```python
from build123d import *

# Parameters (mm, degrees)
IZIM1_R                     = 2
IZIM1_R_2                   = 1.5
Y_KSEKLIK_EKSTR_ZYON1_DEPTH = 1.7
IZIM2_R                     = 2
Y_KSEKLIK_EKSTR_ZYON2_DEPTH = 2.6
IZIM3_W                     = 4.100055298
IZIM3_H                     = 6.25
Y_KSEKLIK_EKSTR_ZYON3_DEPTH = 8.5
IZIM4_W                     = 5.8
IZIM4_H                     = 6.25
Y_KSEKLIK_EKSTR_ZYON4_DEPTH = 0.6
Y_KSEKLIK_EKSTR_ZYON6_DEPTH = 2.54
IZIM6_W                     = 19.85
IZIM6_H                     = 1.7
Y_KSEKLIK_EKSTR_ZYON7_DEPTH = 0.01
IZIM7_W                     = 6.75
IZIM7_H                     = 0.75
KES_EKSTR_ZYON1_DEPTH       = 5.9
KES_EKSTR_ZYON1_DEPTH_BACK  = 0.1
IZIM8_W                     = 0.664910116
IZIM8_H                     = 0.664910116
IZIM11_W                    = 0.65
IZIM11_H                    = 0.6
Y_KSEKLIK_EKSTR_ZYON8_DEPTH = 1
Y_KSEKLIK_EKSTR_ZYON9_DEPTH = 1.5


with BuildPart() as part:
    # Çizim1 → Yükseklik-Ekstrüzyon1 (new body)
    with BuildSketch(Plane.XY):
        with BuildLine():
            Line((-9.925, -11.575), (9.925, -11.575))
            Line((9.925, -11.575), (9.925, 4.275))
            ThreePointArc((9.925, 4.275), (13.575, 7.925), (9.925, 11.575))
            Line((9.925, 11.575), (-9.925, 11.575))
            ThreePointArc((-9.925, 11.575), (-13.575, 7.925), (-9.925, 4.275))
            Line((-9.925, 4.275), (-9.925, -11.575))
        make_face()
        with Locations((9.925, 7.925)):
            Circle(IZIM1_R, mode=Mode.SUBTRACT)
        with Locations((-9.925, 7.925)):
            Circle(IZIM1_R, mode=Mode.SUBTRACT)
        with Locations((7.925, -2.575)):
            Circle(IZIM1_R_2, mode=Mode.SUBTRACT)
        with Locations((-7.925, -2.575)):
            Circle(IZIM1_R_2, mode=Mode.SUBTRACT)
    extrude(amount=Y_KSEKLIK_EKSTR_ZYON1_DEPTH)

    # Çizim2 → Yükseklik-Ekstrüzyon2 (add)
    with BuildSketch(Plane.XY.offset(1.7)):
        with BuildLine():
            Line((-9.925, 11.05), (9.925, 11.05))
            ThreePointArc((9.925, 11.05), (13.05, 7.925), (9.925, 4.8))
            Line((9.925, 4.8), (-9.925, 4.8))
            ThreePointArc((-9.925, 4.8), (-13.05, 7.925), (-9.925, 11.05))
        make_face()
        with Locations((-9.925, 7.925)):
            Circle(IZIM2_R, mode=Mode.SUBTRACT)
        with Locations((9.925, 7.925)):
            Circle(IZIM2_R, mode=Mode.SUBTRACT)
    extrude(amount=Y_KSEKLIK_EKSTR_ZYON2_DEPTH)

    # Çizim3 → Yükseklik-Ekstrüzyon3 (add)
    with BuildSketch(Plane.XY.offset(4.3)):
        with Locations((4.950027649, 7.925)):
            Rectangle(IZIM3_W, IZIM3_H)
        with Locations((-4.950027649, 7.925)):
            Rectangle(IZIM3_W, IZIM3_H)
    extrude(amount=Y_KSEKLIK_EKSTR_ZYON3_DEPTH)

    # Çizim4 → Yükseklik-Ekstrüzyon4 (add)
    with BuildSketch(Plane.XY.offset(4.3)):
        with Locations((0, 7.925)):
            Rectangle(IZIM4_W, IZIM4_H)
    extrude(amount=Y_KSEKLIK_EKSTR_ZYON4_DEPTH)

    # Çizim5 → Yükseklik-Ekstrüzyon6 (add)
    with BuildSketch(Plane(origin=(0, 0, 0), x_dir=(-1, 0, 0), z_dir=(0, 0, -1))):
        Polygon((-1.27, -11.325), (-1.27, -9.285), (-1.52, -9.035), (-3.56, -9.035), (-3.81, -9.285), (-3.81, -11.325), (-3.56, -11.575), (-1.52, -11.575), align=None)
        Polygon((1.27, -9.285), (1.02, -9.035), (-1.02, -9.035), (-1.27, -9.285), (-1.27, -11.325), (-1.02, -11.575), (1.02, -11.575), (1.27, -11.325), align=None)
        Polygon((1.52, -9.035), (1.27, -9.285), (1.27, -11.325), (1.52, -11.575), (3.56, -11.575), (3.81, -11.325), (3.81, -9.285), (3.56, -9.035), align=None)
    extrude(amount=Y_KSEKLIK_EKSTR_ZYON6_DEPTH)

    # Çizim6 → Yükseklik-Ekstrüzyon7 (add)
    with BuildSketch(Plane.XZ.offset(11.575)):
        with Locations((0, 0.85)):
            Rectangle(IZIM6_W, IZIM6_H)
    extrude(amount=Y_KSEKLIK_EKSTR_ZYON7_DEPTH)

    # Çizim7 → Kes-Ekstrüzyon1 (cut, two sides)
    with BuildSketch(Plane.ZY.offset(-2.9)) as kes_ekstr_zyon1_sk:
        with Locations((8.275, 7.925)):
            Rectangle(IZIM7_W, IZIM7_H)
    extrude(amount=KES_EKSTR_ZYON1_DEPTH, mode=Mode.SUBTRACT)
    extrude(kes_ekstr_zyon1_sk.sketch, amount=-KES_EKSTR_ZYON1_DEPTH_BACK, mode=Mode.SUBTRACT)

    # Süpür1: sweep along a path in Çizim9
    with BuildLine(Plane(origin=(0, 0, 0), x_dir=(0, 0, -1), z_dir=(1, 0, 0))) as s_p_r1_path:
        Line((2.54, -10.305), (4.04, -10.305))
        ThreePointArc((4.04, -10.305), (4.393553391, -10.158553391), (4.54, -9.805))
        Line((4.54, -9.805), (4.54, -3.305))
    # Çizim8 → Süpür1 (sweep)
    with BuildSketch(Plane(origin=(0, 0, -2.54), x_dir=(-1, 0, 0), z_dir=(0, 0, -1))):
        with Locations((2.54, -10.305)):
            Rectangle(IZIM8_W, IZIM8_H)
        with Locations((0, -10.305)):
            Rectangle(IZIM8_W, IZIM8_H)
        with Locations((-2.54, -10.305)):
            Rectangle(IZIM8_W, IZIM8_H)
    sweep(path=s_p_r1_path.line)

    # Çizim11 → Yükseklik-Ekstrüzyon8 (add)
    with BuildSketch(Plane.XY.offset(1.7)):
        with Locations((-2.54, -10.305)):
            Rectangle(IZIM11_W, IZIM11_H)
        with Locations((0, -10.305)):
            Rectangle(IZIM11_W, IZIM11_H)
        with Locations((2.54, -10.305)):
            Rectangle(IZIM11_W, IZIM11_H)
    extrude(amount=Y_KSEKLIK_EKSTR_ZYON8_DEPTH)

    # Çizim12 → Yükseklik-Ekstrüzyon9 (add)
    with BuildSketch(Plane(origin=(0, 0, 0), x_dir=(-1, 0, 0), z_dir=(0, 0, -1))):
        Polygon((-3.925, -2.575), (-3.925, -0.075), (-0.175, -0.075), (-0.175, -5.075), (-3.925, -5.075), align=None)
    extrude(amount=Y_KSEKLIK_EKSTR_ZYON9_DEPTH)


solid = part.part
```
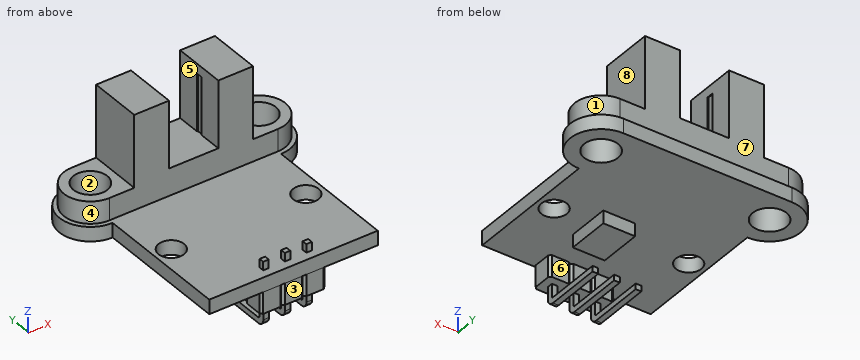
For this review, take the finished solid that the model builds, in its own axes (mm). Face numbers are marked on the shaded views. A direction names the side the tool comes from. Round coordinates to 2 decimals unless told otherwise and drop trailing zeros. Order: outer loops, then holes, each group sorted by start corner. A loop starts at its lowest first (then second) coordinate and runs counter-clockwise, first axis right, second up.
Q1. Insertion check: P1, Ø3, axis at y = 7.5, z = 7.5, coming from the +X side; P2, Ø3.5, axis at x = 3.5, z = 5, coming from the -Y side; P3, Ø5, axis at x = 3, y = 0.5, coming from the +Z side. Each pin has a flat end and moves straight along its axis. Give the tip position at first contact, or say it passes through.
Findings below:
P1: stops at x = 7
P2: stops at y = 4.8
P3: stops at z = 1.7
Q2. We need section C-C, the plane y = -8.5. Give the boundary of the cut face in (x, z) (3 decimals).
Findings below:
outline: (-9.925, 0) - (9.925, 0) - (9.925, 1.7) - (-9.925, 1.7) - close; (-2.872, -4.872) - (-2.208, -4.872) - (-2.208, -4.208) - (-2.872, -4.208) - close; (-0.332, -4.872) - (0.332, -4.872) - (0.332, -4.208) - (-0.332, -4.208) - close; (2.208, -4.872) - (2.872, -4.872) - (2.872, -4.208) - (2.208, -4.208) - close
Q3. We need section D-D, the plane z = -3. Give the boundary of the cut face in (x, y), plus the area to 3 significant figures.
Findings below:
outline: (-2.87, -10.64) - (-2.21, -10.64) - (-2.21, -9.97) - (-2.87, -9.97) - close; (-0.33, -10.64) - (0.33, -10.64) - (0.33, -9.97) - (-0.33, -9.97) - close; (2.21, -10.64) - (2.87, -10.64) - (2.87, -9.97) - (2.21, -9.97) - close
area: 1.33 mm2
Q4. Wall thickness on line 1 (X direction, y = -2.5, z = 0.25) (3 decimals); line 2 (X direction, y = -1.5, z = 1) (3 decimals); line 3 (Y direction, x = -8.75, z = 0.5) (3 decimals): over which ranges is each line inside the solid? List them lowest first.
Findings below:
line 1: x = -9.925 to -9.423, -6.427 to 6.427, 9.423 to 9.925
line 2: x = -9.925 to -8.971, -6.879 to 6.879, 8.971 to 9.925
line 3: y = -11.585 to -3.828, -1.322 to 6.307, 9.543 to 11.575
Q5. Machinability: for the marked faces 4, 5, 6, 7 and 8, which of the approach directions +Z, -Z, +X, -X, +Y, -Y give a long, thin tool a straight path to every point of the face, cutting with its end or side? Answer none if there is none.
Findings below:
face 4: +Z, -X
face 5: +Z, +Y, -Y
face 6: +X, -X
face 7: +Z, +X, -X, +Y
face 8: +Z, +X, +Y, -Y
Q6. We need section B-B, the plane z = 6.5. Give the boundary of the cut face in (x, y).
Findings below:
outline: (-7, 4.8) - (-2.9, 4.8) - (-2.9, 7.55) - (-3, 7.55) - (-3, 8.3) - (-2.9, 8.3) - (-2.9, 11.05) - (-7, 11.05) - close; (2.9, 4.8) - (7, 4.8) - (7, 11.05) - (2.9, 11.05) - (2.9, 8.3) - (3, 8.3) - (3, 7.55) - (2.9, 7.55) - close
Q7. We need section A-A, the plane z = 2.25. Give the boundary of the cut face in (x, y) (3 decimals).
Findings below:
outline: (-9.925, 4.8) - (9.925, 4.8) arc R3.125 ccw to (9.925, 11.05) - (-9.925, 11.05) arc R3.125 ccw to start; (-2.865, -10.605) - (-2.215, -10.605) - (-2.215, -10.005) - (-2.865, -10.005) - close; (-0.325, -10.605) - (0.325, -10.605) - (0.325, -10.005) - (-0.325, -10.005) - close; (2.215, -10.605) - (2.865, -10.605) - (2.865, -10.005) - (2.215, -10.005) - close; hole circle Ø4 at (-9.925, 7.925); hole circle Ø4 at (9.925, 7.925)
Q8. Mouldability with a two-part tool opening along Y and no side actions: class the marked faces 1, 2 and 3 as pulls with the +Y half, pulls with the -Y half, needs draft (parallel to the pull), parting line crosses it, or undercut.
Findings below:
face 1: parting line crosses it
face 2: undercut
face 3: pulls with the -Y half
